Work out the finished part from the listing and answer in its coordinate system (mm). A direction names the side the tool comes from. Give positions to 0.01 mm unless a question says otherwise; leave off trailing zeros. Write each loop counter-clockwise with the first axis right and the second up, starting at its lowest first coordinate (ties: lowest second). Pieces come first, ordered by that corner, then holes.
1) Given pin 1 Ø8 at (x, z) = (-9, 427.5) entering from -Y; pin 2 Ø1.5 at (x, z) = (10.5, 236.5) entering from -Y; pin 3 Ø1.5 at (x, y) = (7.5, -229.5) entering from +Z, each flat-ended and moving along its own axis, determine where each tip first touches the part or whether it passes through.
2) Find section A-A (x = -5.5). Determine the outline of the cut face in (y, z), plus the area to 3 significant figures.
3) Determine the mould class of faces 4 (the face through (-3.62, -499.903, 562.191)), 5 (the face through (14.79, -12.33, 0.15)), 6 (the face through (12.87, -169.43, -5.34)) for opening direction X: pulls with the +X half, pulls with the -X half, needs draft (parallel to the pull), parting line crosses it, or undercut.
4) A tool of negligible diameter and unlimited length cuts with its end or side. For faces 1 (the face through (-1.814, -469.787, 562.191)), 2 (the face through (-9, -495, 963)), 3 (the face through (15.929, -169.43, 5.016)), from which of +Z, -Z, +X, -X, +Y, -Y can it reach the whole face along a straight path? Write none if from no direction.
5) Straight lines are drawn through the part: probe 1 along Z at (x, y) = (-9, -216); probe 2 along X at (y, z) = (-246, 0). For each, find the intervals that lie inside material, in ascending order.
6) Find section C-C (z = 720). Determine the outline of the cut face in (x, y).
7) Find section B-B (y = -94). Determine the outline of the cut face in (x, z).
```python
from build123d import *

# Parameters (mm, degrees)
F1_R          = 16.7
F1_R_2        = 13.932
F4_DEPTH      = 16.7010001
F4_DEPTH_BACK = 963.001


with BuildPart() as f2:
    # F2: sweep along a path in F0
    with BuildLine(Plane.YZ) as f2_path:
        Line((0, 0), (-333.6, 0))
        ThreePointArc((-333.6, 0), (-439.666017178, 43.933982822), (-483.6, 150))
        Line((-483.6, 150), (-483.6, 963))
    # F1 (on Front) → F2 (sweep)
    with BuildSketch(Plane.XZ):
        Circle(F1_R)
        Circle(F1_R_2, mode=Mode.SUBTRACT)
    sweep(path=f2_path.line)

    # F3 (on Top) → F4 (cut, two sides)
    with BuildSketch(Plane.XY) as f4_sk:
        Polygon((-16.7, 0), (0, 0), (-16.7, 2.6450201534), align=None)
        Polygon((16.7, 0), (0, 0), (-16.7, 0), (-16.7, -5.2900403068), (12.9306502179, -0.5970063556), (16.7, -24.395744252), (16.7, -5.4741381354), (16.7, -2.6450201534), align=None)
    extrude(amount=-F4_DEPTH, mode=Mode.SUBTRACT)
    extrude(f4_sk.sketch, amount=F4_DEPTH_BACK, mode=Mode.SUBTRACT)


solid = f2.part
```
Results:
1. pin 1: stops at y = -499.53
1. pin 2: stops at y = -497.16
1. pin 3: stops at z = 15.28
2. outline: (-499.37, 150) arc R165.77 ccw to (-333.6, -15.77) - (-3.52, -15.77) - (-3.52, -12.8) - (-333.6, -12.8) arc R162.8 cw to (-496.4, 150) - (-496.4, 963) - (-499.37, 963) - close; (-470.8, 150) arc R137.2 ccw to (-333.6, 12.8) - (-3.52, 12.8) - (-3.52, 15.77) - (-333.6, 15.77) arc R134.23 cw to (-467.83, 150) - (-467.83, 963) - (-470.8, 963) - close
2. area: 8,180 mm2
3. face 4: parting line crosses it
3. face 5: pulls with the +X half
3. face 6: undercut
4. face 1: +Z
4. face 2: +Z, +X, -X, +Y, -Y
4. face 3: +Y
5. probe 1: z = -14.07 to -10.63, 10.63 to 14.07
5. probe 2: x = -16.7 to -13.93, 13.93 to 16.7
6. outline: circle Ø33.4 at (0, -483.6); hole circle Ø27.86 at (0, -483.6)
7. outline: circle Ø33.4 at (0, 0); hole circle Ø27.86 at (0, 0)
